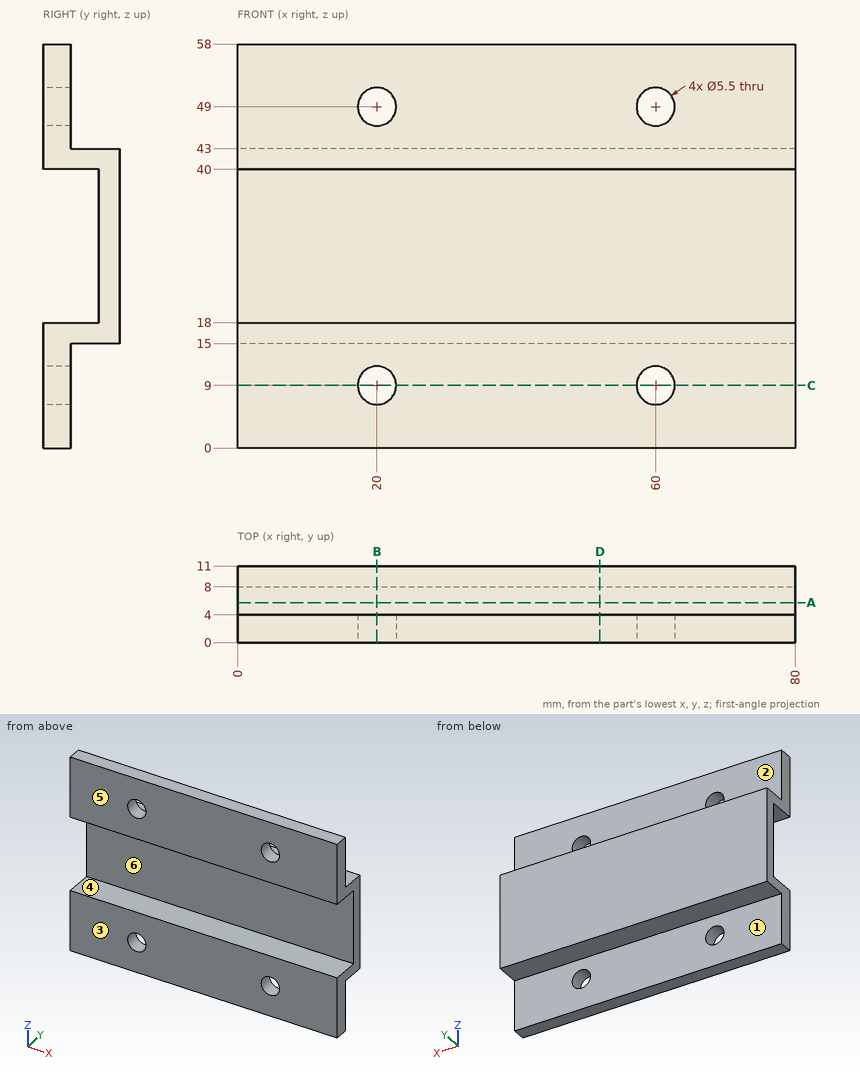
Input: dimensioned drawing with shaded views. Units: mm. Origin: part minimum x, y, z. A direction names the side the tool comes from. Give positions to 0.01 mm unless a question says otherwise; leave off trailing zeros. Write each loop counter-clockwise with the first axis right and the second up, starting at its lowest first coordinate (ties: lowest second). Pieces come first, ordered by that corner, then holes.
Q1. Section D-D, the plane x = 52. Output: boundary loops of the cut face in (y, z), plus the area to 3 significant figures.
Q2. Section A-A, the plane y = 5.75. Output: boundary loops of the cut face in (x, z), plus the area to 3 significant figures.
Q3. First-contact query: P1, Ø12, axis at x = 51, z = 54, coming from the +Y side; P2, Ø3.5, axis at x = 60, z = 49, coming from the +Y side; P3, Ø2.5, axis at x = 38.5, y = 5.5, coming from the +Z side. Flat tips, straight axial feed; report the tip coordinate or a pass-through.
Q4. Section C-C, the plane z = 9. Output: boundary loops of the cut face in (x, y), plus the area to 3 significant figures.
Q5. Set-up query: the marked faces 1, 2 and 3. Return all of +Z, -Z, +X, -X, +Y, -Y with unobstructed straight access to the full face (end or side cutting, diameter ignored); none if empty.
Q6. Section B-B, the plane x = 20. Output: boundary loops of the cut face in (y, z), plus the area to 3 significant figures.
Q7. Material intervals for probe 1 along Z at (x, y) = (20, 2.45); probe 2 along X at (y, z) = (1.95, 49); probe 3 along X at (y, z) = (2.25, 48), sorted ascending.
Q8. Pull-direction query (Z, two-part tool) for the marked faces 4, 5 and 6; classes: pulls with the +Z half, pulls with the -Z half, needs draft (parallel to the pull), parting line crosses it, or undercut.
Filled in:
1. outline: (0, 0) - (4, 0) - (4, 15) - (11, 15) - (11, 43) - (4, 43) - (4, 58) - (0, 58) - (0, 40) - (8, 40) - (8, 18) - (0, 18) - close
1. area: 252 mm2
2. outline: (0, 15) - (80, 15) - (80, 18) - (0, 18) - close; (0, 40) - (80, 40) - (80, 43) - (0, 43) - close
2. area: 480 mm2
3. P1: stops at y = 4
3. P2: passes through
3. P3: stops at z = 43
4. outline: (0, 0) - (17.25, 0) - (17.25, 4) - (0, 4) - close; (22.75, 0) - (57.25, 0) - (57.25, 4) - (22.75, 4) - close; (62.75, 0) - (80, 0) - (80, 4) - (62.75, 4) - close
4. area: 276 mm2
5. face 1: -Z, +X, -X, +Y
5. face 2: +Z, +X, -X, +Y
5. face 3: +Z, -Z, +X, -X, -Y
6. outline: (0, 0) - (4, 0) - (4, 6.25) - (0, 6.25) - close; (0, 11.75) - (4, 11.75) - (4, 15) - (11, 15) - (11, 43) - (4, 43) - (4, 46.25) - (0, 46.25) - (0, 40) - (8, 40) - (8, 18) - (0, 18) - close; (0, 51.75) - (4, 51.75) - (4, 58) - (0, 58) - close
6. area: 208 mm2
7. probe 1: z = 0 to 6.25, 11.75 to 18, 40 to 46.25, 51.75 to 58
7. probe 2: x = 0 to 17.25, 22.75 to 57.25, 62.75 to 80
7. probe 3: x = 0 to 17.44, 22.56 to 57.44, 62.56 to 80
8. face 4: undercut
8. face 5: needs draft
8. face 6: undercut
